Can you work these out from the model? Positions are in its coordinate system, mm. Give positions to 0.01 mm unless a question says otherwise; leave off trailing zeros. Write each loop counter-clockwise with the first axis right and the second up, starting at its lowest first coordinate (ties: lowest second). Pieces come first, ordered by that corner, then holes. Notation, with made-up numbers: M 40,-37 L 71,-37 A23 ccw 71,-22 Z; hole C -11.5,5 d3. An arc over 180 degrees is marked long. Write each question's results on one line, items separated by ' | '.
from build123d import *

# Parameters (mm, degrees)
BOSS_EXTRUDE1_DEPTH      = 254
BOSS_EXTRUDE1_DEPTH_BACK = 185.42
SKETCH1_W                = 12.7
SKETCH1_H                = 12.7
SKETCH1_W_2              = 9.525
SKETCH1_H_2              = 9.525
CUT_EXTRUDE1_DEPTH       = 255.158700422
CUT_EXTRUDE1_DEPTH_BACK  = 255.158700422


with BuildPart() as part:
    # Sketch1 → Boss-Extrude1 (new, two sides: drawn at the far end of the back side and taken through both)
    with BuildSketch(Plane(origin=(0, 0, 0), x_dir=(0, 0, -1), z_dir=(1, 0, 0)).offset(-BOSS_EXTRUDE1_DEPTH_BACK)):
        Rectangle(SKETCH1_W, SKETCH1_H)
        Rectangle(SKETCH1_W_2, SKETCH1_H_2, mode=Mode.SUBTRACT)
    extrude(amount=BOSS_EXTRUDE1_DEPTH + BOSS_EXTRUDE1_DEPTH_BACK)

    # Sketch2 → Cut-Extrude1 (cut, two sides: drawn at the far end of the back side and taken through both)
    with BuildSketch(Plane(origin=(0, 0, 0), x_dir=(1, 0, 0), z_dir=(0, 1, 0)).offset(-CUT_EXTRUDE1_DEPTH_BACK)):
        Polygon((-185.42, -6.35), (-174.250456919, 6.961343094), (-183.078216502, 14.368712905), (-194.247759583, 1.057369811), align=None)
    extrude(amount=CUT_EXTRUDE1_DEPTH + CUT_EXTRUDE1_DEPTH_BACK, mode=Mode.SUBTRACT)


solid = part.part
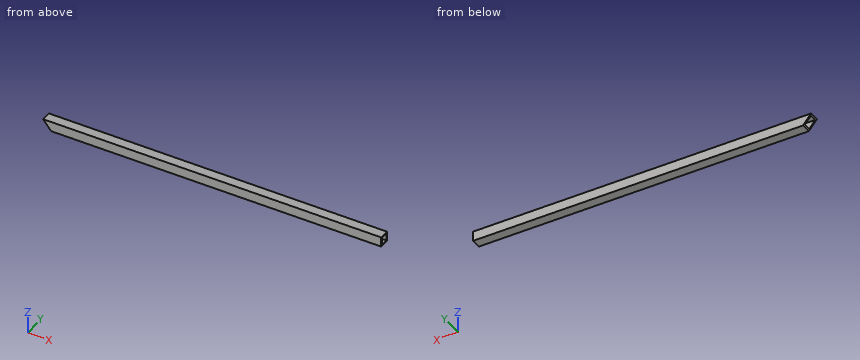
Item 1: I want a section at B-B, the plane z = 0.5. Please give me the cut outline in (x, y).
Geometry says:
outline: M -180.51,-6.35 L 254,-6.35 L 254,-4.76 L -180.51,-4.76 Z; M -180.51,4.76 L 254,4.76 L 254,6.35 L -180.51,6.35 Z
Item 2: I'm going to push a flat-ended pin straight in: pin 1 (3 mm diameter, centred on y = 2, z = -4, fed in from -X). Where does the tip first touch, or does it pass through?
Geometry says:
pin 1: stops at x = -176.1
Item 3: If I drill on line 1 (Z direction, x = 98, y = 4); line 2 (X direction, y = 6, z = -3.75), over which ranges is the centre line in solid material (lowest first)? Write a range as from..to.
Geometry says:
line 1: z = -6.35..-4.76, 4.76..6.35 | line 2: x = -176.95..254
Item 4: I want a section at A-A, the plane y = -2. Please give me the cut outline in (x, z), and give its area (3 significant figures).
Geometry says:
outline: M -185.42,6.35 L -184.09,4.76 L 254,4.76 L 254,6.35 Z; M -176.1,-4.76 L -174.76,-6.35 L 254,-6.35 L 254,-4.76 Z | area: 1,380 mm2
Item 5: I want a section at C-C, the plane x = 179. Please give me the cut outline in (y, z), and give its area (3 significant figures).
Geometry says:
outline: M -6.35,-6.35 L 6.35,-6.35 L 6.35,6.35 L -6.35,6.35 Z; hole M -4.76,-4.76 L 4.76,-4.76 L 4.76,4.76 L -4.76,4.76 Z | area: 70.6 mm2
